The model under review builds one solid part; all positions refer to its coordinate system, in mm. Face numbers are marked on the shaded views. A direction names the side the tool comes from. Round coordinates to 2 decimals unless told otherwise and drop trailing zeros. Write each loop counter-clockwise with the first axis right and the second up, starting at its lowest first coordinate (ties: lowest second). Pieces come first, ordered by that corner, then holes. Notation, with made-up numbers: (34, -19) -> (82, -19) arc R22 ccw to (82, 9) -> close; hole circle Ø10 at (-16.75, -6.75). An arc over 180 degrees is marked (long way). Answer in a Markdown table with one row per item. Add a question column.
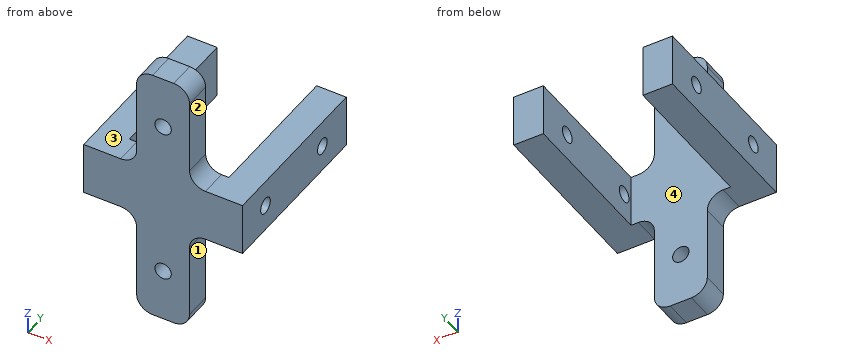
```python
from build123d import *

# Parameters (mm, degrees)
SKETCH1_W                      = 30
SKETCH1_H                      = 10
BOSS_EXTRUDE1_DEPTH            = 5
SKETCH2_W                      = 5.6
SKETCH2_H                      = 10
BOSS_EXTRUDE2_DEPTH            = 27.3
CUT_EXTRUDE1_REACH             = 49.484
SKETCH3_R                      = 1.5
CUT_EXTRUDE1_DIRECTION_2_REACH = 49.484
SKETCH4_W                      = 10
SKETCH4_H                      = 5
BOSS_EXTRUDE3_DEPTH            = 20
SKETCH5_W                      = 10
SKETCH5_H                      = 5
BOSS_EXTRUDE4_DEPTH            = 20
SKETCH6_R                      = 1.55
CUT_EXTRUDE2_DEPTH             = 62.172994556
FILLET1_R                      = 3


with BuildPart() as part:
    # Sketch1 → Boss-Extrude1 (new body)
    with BuildSketch(Plane(origin=(0, 0, 0), x_dir=(1, 0, 0), z_dir=(0, 1, 0))):
        with Locations((-16.432463279, 19.820146309)):
            Rectangle(SKETCH1_W, SKETCH1_H)
    extrude(amount=BOSS_EXTRUDE1_DEPTH)

    # Sketch2 → Boss-Extrude2 (add)
    with BuildSketch(Plane(origin=(0, 5, 0), x_dir=(1, 0, 0), z_dir=(0, 1, 0))):
        with Locations((-28.632463279, 19.820146309)):
            Rectangle(SKETCH2_W, SKETCH2_H)
        with Locations((-4.232463279, 19.820146309)):
            Rectangle(SKETCH2_W, SKETCH2_H)
    extrude(amount=BOSS_EXTRUDE2_DEPTH)

    # Cut-Extrude1: up to this face of the body (flat: up to its plane)
    cut_extrude1_end = Plane(part.part.faces().sort_by_distance((-31.432463279, 16.15, -19.820146309))[0])
    # Sketch3 → Cut-Extrude1 (cut, up to the picked face)
    with BuildSketch(Plane(origin=(-25.832463279, 0, 0), x_dir=(0, 0, -1), z_dir=(1, 0, 0)), mode=Mode.PRIVATE) as cut_extrude1_sk1:
        with Locations((19.820146309, 7.15)):
            Circle(SKETCH3_R)
    cut_extrude1_tool1 = split(extrude(cut_extrude1_sk1.sketch, amount=-CUT_EXTRUDE1_REACH, mode=Mode.PRIVATE), bisect_by=cut_extrude1_end, keep=Keep.BOTH, mode=Mode.PRIVATE)
    # Sketch3 → Cut-Extrude1 (cut, up to the picked face)
    with BuildSketch(Plane(origin=(-25.832463279, 0, 0), x_dir=(0, 0, -1), z_dir=(1, 0, 0)), mode=Mode.PRIVATE) as cut_extrude1_sk2:
        with Locations((19.820146309, 24.85)):
            Circle(SKETCH3_R)
    cut_extrude1_tool2 = split(extrude(cut_extrude1_sk2.sketch, amount=-CUT_EXTRUDE1_REACH, mode=Mode.PRIVATE), bisect_by=cut_extrude1_end, keep=Keep.BOTH, mode=Mode.PRIVATE)
    add(cut_extrude1_tool1.solids().sort_by(Axis((-25.832463, 7.15, -19.820146), (-1, 0, 0)))[0], mode=Mode.SUBTRACT)
    add(cut_extrude1_tool2.solids().sort_by(Axis((-25.832463, 24.85, -19.820146), (-1, 0, 0)))[0], mode=Mode.SUBTRACT)

    # Cut-Extrude1 direction 2: up to this face of the body (flat: up to its plane)
    cut_extrude1_direction_2_end = Plane(part.part.faces().sort_by_distance((-1.432463279, 16.15, -19.820146309))[0])
    # Sketch3 → Cut-Extrude1 direction 2 (cut, up to the picked face)
    with BuildSketch(Plane(origin=(-25.832463279, 0, 0), x_dir=(0, 0, -1), z_dir=(1, 0, 0)), mode=Mode.PRIVATE) as cut_extrude1_direction_2_sk1:
        with Locations((19.820146309, 7.15)):
            Circle(SKETCH3_R)
    cut_extrude1_direction_2_tool1 = split(extrude(cut_extrude1_direction_2_sk1.sketch, amount=CUT_EXTRUDE1_DIRECTION_2_REACH, mode=Mode.PRIVATE), bisect_by=cut_extrude1_direction_2_end, keep=Keep.BOTH, mode=Mode.PRIVATE)
    # Sketch3 → Cut-Extrude1 direction 2 (cut, up to the picked face)
    with BuildSketch(Plane(origin=(-25.832463279, 0, 0), x_dir=(0, 0, -1), z_dir=(1, 0, 0)), mode=Mode.PRIVATE) as cut_extrude1_direction_2_sk2:
        with Locations((19.820146309, 24.85)):
            Circle(SKETCH3_R)
    cut_extrude1_direction_2_tool2 = split(extrude(cut_extrude1_direction_2_sk2.sketch, amount=CUT_EXTRUDE1_DIRECTION_2_REACH, mode=Mode.PRIVATE), bisect_by=cut_extrude1_direction_2_end, keep=Keep.BOTH, mode=Mode.PRIVATE)
    add(cut_extrude1_direction_2_tool1.solids().sort_by(Axis((-25.832463, 7.15, -19.820146), (1, 0, 0)))[0], mode=Mode.SUBTRACT)
    add(cut_extrude1_direction_2_tool2.solids().sort_by(Axis((-25.832463, 24.85, -19.820146), (1, 0, 0)))[0], mode=Mode.SUBTRACT)

    # Sketch4 → Boss-Extrude3 (add)
    with BuildSketch(Plane(origin=(0, 0, -24.820146309), x_dir=(-1, 0, 0), z_dir=(0, 0, -1))):
        with Locations((16.432463279, 2.5)):
            Rectangle(SKETCH4_W, SKETCH4_H)
    extrude(amount=BOSS_EXTRUDE3_DEPTH)

    # Sketch5 → Boss-Extrude4 (add)
    with BuildSketch(Plane.XY.offset(-14.820146309)):
        with Locations((-16.432463279, 2.5)):
            Rectangle(SKETCH5_W, SKETCH5_H)
    extrude(amount=BOSS_EXTRUDE4_DEPTH)

    # Sketch6 → Cut-Extrude2 (cut, through all)
    with BuildSketch(Plane(origin=(0, 5, 0), x_dir=(1, 0, 0), z_dir=(0, 1, 0))):
        with Locations(Location((-16.432463279, 34.885731697, 0), (0, 0, 270))):
            Circle(SKETCH6_R)
        with Locations(Location((-16.432463279, 4.754560921, 0), (0, 0, 270))):
            Circle(SKETCH6_R)
    extrude(amount=-CUT_EXTRUDE2_DEPTH, mode=Mode.SUBTRACT)

    # Fillet1
    fillet1_edges = [part.edges().sort_by_distance(p)[0] for p in [
        (-21.432463279, 2.5, -24.820146309),
        (-21.432463279, 2.5, -44.820146309),
        (-11.432463279, 2.5, -44.820146309),
        (-11.432463279, 2.5, -24.820146309),
        (-11.432463279, 2.5, -14.820146309),
        (-21.432463279, 2.5, -14.820146309),
        (-11.432463279, 2.5, 5.179853691),
        (-21.432463279, 2.5, 5.179853691),
    ]]
    fillet(fillet1_edges, radius=FILLET1_R)


solid = part.part
```
1. Add section B-B on y = 24.85. Write out the cut boundary in (x, z), plus the area to 3 significant figures.
2. Add section D-D on z = -20.5. Write out the cut boundary in (x, y).
3. Add section C-C on x = -4.25. Write out the cut boundary in (y, z).
4. Tool access review of the marked faces 1, 2, 3 and 4: name each direction out of +Z, -Z, +X, -X, +Y, -Y from which nothing blocks a thin tool from reaching the whole face with its end or side.
5. For L1, parallel to X at y = 12, z = -23; L2, parallel to Z at x = -5.1, y = 24.85; L3, parallel to Y at x = -8, z = -21, list the stretches that pass through material, from the lowest coordinate up.
6. Add section A-A on y = 11.5. Write out the cut boundary in (x, z), plus the area to 3 significant figures.
7. Insertion check: pin 1 Ø10 at (x, y) = (-24, 17) entering from +Z; pin 2 Ø1 at (x, y) = (-6, 22) entering from -Z; pin 3 Ø5.5 at (y, z) = (2, -5.5) entering from +X. Each pin has a flat end and moves straight along its axis. Give the tip position at first contact, or say it passes through.
Filled in:
| question | item | result |
|---|---|---|
| 1 | outline | (-31.43, -24.82) -> (-25.83, -24.82) -> (-25.83, -21.32) -> (-31.43, -21.32) -> close; (-31.43, -18.32) -> (-25.83, -18.32) -> (-25.83, -14.82) -> (-31.43, -14.82) -> close; (-7.03, -24.82) -> (-1.43, -24.82) -> (-1.43, -21.32) -> (-7.03, -21.32) -> close; (-7.03, -18.32) -> (-1.43, -18.32) -> (-1.43, -14.82) -> (-7.03, -14.82) -> close |
| 1 | area | 78.4 mm² |
| 2 | outline | (-31.43, 0) -> (-1.43, 0) -> (-1.43, 5.81) -> (-7.03, 5.81) -> (-7.03, 5) -> (-25.83, 5) -> (-25.83, 5.81) -> (-31.43, 5.81) -> close; (-31.43, 8.49) -> (-25.83, 8.49) -> (-25.83, 23.51) -> (-31.43, 23.51) -> close; (-31.43, 26.19) -> (-25.83, 26.19) -> (-25.83, 32.3) -> (-31.43, 32.3) -> close; (-7.03, 8.49) -> (-1.43, 8.49) -> (-1.43, 23.51) -> (-7.03, 23.51) -> close; (-7.03, 26.19) -> (-1.43, 26.19) -> (-1.43, 32.3) -> (-7.03, 32.3) -> close |
| 3 | outline | (0, -24.82) -> (32.3, -24.82) -> (32.3, -14.82) -> (0, -14.82) -> close; hole circle Ø3 at (7.15, -19.82); hole circle Ø3 at (24.85, -19.82) |
| 4 | face 1 | -Z, +X, +Y, -Y |
| 4 | face 2 | +Z, +X, +Y, -Y |
| 4 | face 3 | +Z, -X, +Y, -Y |
| 4 | face 4 | +Z, -Z, +Y |
| 5 | L1 | -31.43 to -25.83, -7.03 to -1.43 |
| 5 | L2 | -24.82 to -21.32, -18.32 to -14.82 |
| 5 | L3 | 0 to 5 |
| 6 | outline | (-31.43, -24.82) -> (-25.83, -24.82) -> (-25.83, -14.82) -> (-31.43, -14.82) -> close; (-7.03, -24.82) -> (-1.43, -24.82) -> (-1.43, -14.82) -> (-7.03, -14.82) -> close |
| 6 | area | 112 mm² |
| 7 | pin 1 | z = -14.82 |
| 7 | pin 2 | z = -24.82 |
| 7 | pin 3 | x = -11.43 |
